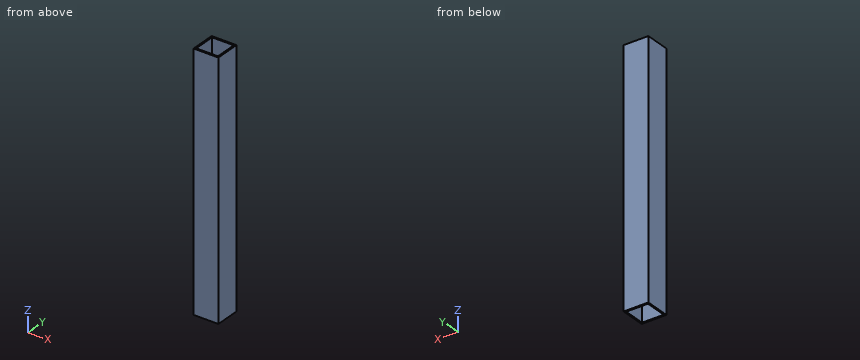
from build123d import *

# Parameters (mm, degrees)
EXTRUDE1_DEPTH      = 236.728
EXTRUDE1_DEPTH_BACK = 19.05
SKETCH1_W           = 25.4
SKETCH1_H           = 25.4
SKETCH1_W_2         = 22.225
SKETCH1_H_2         = 22.225


with BuildPart() as part:
    # Sketch1 → Extrude1 (new, two sides: drawn at the far end of the back side and taken through both)
    with BuildSketch(Plane.XY.offset(-EXTRUDE1_DEPTH_BACK)):
        with Locations((0, -15.875)):
            Rectangle(SKETCH1_W, SKETCH1_H)
        with Locations((0, -15.875)):
            Rectangle(SKETCH1_W_2, SKETCH1_H_2, mode=Mode.SUBTRACT)
    extrude(amount=EXTRUDE1_DEPTH + EXTRUDE1_DEPTH_BACK)


solid = part.part
Geometry check sheet. Reference: the model listing, model coordinates, mm. Give positions to 0.01 mm unless a question says otherwise; leave off trailing zeros. Loops run counter-clockwise (first coordinate to the right, second up) from the corner with the lowest first, then second, coordinate; pieces in that order, holes last. Notation, with made-up numbers: (38, 63) -> (49, 63) arc R28 cw to (49, 91) -> close; hole circle Ø1 at (-33.75, 37.5). An arc over 180 degrees is marked (long way). Answer in a Markdown table with one row per item. Add a question column.
1) Cross-section at A-A on y = -14. Record the boundary of the cut face in (x, z).
2) Gauge pin test, flat end, axial feed: P1, Ø5, axis at x = -4, y = -23, coming from the -Z side. Record the tip position at first contact, or that the pin passes through.
3) Material ranges on probe 1 along X at (y, z) = (-9.25, 74); probe 2 along Y at (x, z) = (5.5, 191) (1 decimal), recorded low to high. Write a range as from..to.
4) Cross-section at C-C on z = 181. Record the boundary of the cut face in (x, y) (1 decimal), and give its area (3 significant figures).
Outcome:
| question | item | result |
|---|---|---|
| 1 | outline | (-12.7, -19.05) -> (-11.11, -19.05) -> (-11.11, 236.73) -> (-12.7, 236.73) -> close; (11.11, -19.05) -> (12.7, -19.05) -> (12.7, 236.73) -> (11.11, 236.73) -> close |
| 2 | P1 | passes through |
| 3 | probe 1 | x = -12.7..-11.11, 11.11..12.7 |
| 3 | probe 2 | y = -28.6..-27, -4.8..-3.2 |
| 4 | outline | (-12.7, -28.6) -> (12.7, -28.6) -> (12.7, -3.2) -> (-12.7, -3.2) -> close; hole (-11.1, -27) -> (11.1, -27) -> (11.1, -4.8) -> (-11.1, -4.8) -> close |
| 4 | area | 151 mm^2 |
